Autodesk Inventor part; units mm, degrees
ref_plane "to_blackets_XY" through (0, 0, -4.5) normal (1, 0, 0) x (0, 0, -1)
ref_plane "to_blackets_YZ" through (0, 0, -4.5) normal (0, 0, -1) x (0, 1, 0)
ref_plane "to_blackets_ZX" through (0, 0, -4.5) normal (0, 1, 0) x (1, 0, 0)
sketch "_____1" plane through (0, 0, 0) normal (0, 0, 1) x (1, 0, 0)
  line L0 (-4.1, 2.7981) -> (-4.1, -2.7981)
  arc A0 (-4.1, -2.7981) -> (-4.0176, -2.9599) centre (-3.9, -2.7981) ccw
  line L1 (-4.0176, -2.9599) -> (-1.2622, -4.9618)
  arc A1 (-1.2622, -4.9618) -> (-1.1446, -5) centre (-1.1446, -4.8) ccw
  line L2 (-1.1446, -5) -> (-1, -5)
  arc A2 (-1, -5) -> (-0.8, -4.8) centre (-1, -4.8) ccw
  line L3 (-0.8, -4.8) -> (-0.8, -3)
  arc A3 (-0.7, -2.9) -> (-0.8, -3) centre (-0.7, -3) ccw
  line L4 (-0.7, -2.9) -> (-0.2, -2.9)
  arc A4 (-0.2, -2.9) -> (0, -2.7) centre (-0.2, -2.7) ccw
  line L5 (0, -2.7) -> (0, 2.7)
  arc A5 (0, 2.7) -> (-0.2, 2.9) centre (-0.2, 2.7) ccw
  line L6 (-0.2, 2.9) -> (-0.7, 2.9)
  arc A6 (-0.8, 3) -> (-0.7, 2.9) centre (-0.7, 3) ccw
  line L7 (-0.8, 3) -> (-0.8, 4.8)
  arc A7 (-0.8, 4.8) -> (-1, 5) centre (-1, 4.8) ccw
  line L8 (-1, 5) -> (-1.1446, 5)
  arc A8 (-1.1446, 5) -> (-1.2622, 4.9618) centre (-1.1446, 4.8) ccw
  line L9 (-1.2622, 4.9618) -> (-4.0176, 2.9599)
  arc A9 (-4.0176, 2.9599) -> (-4.1, 2.7981) centre (-3.9, 2.7981) ccw
extrude "Extrusion1" add sketch "_____1" against normal blind 14
sketch "_____2" plane through (0, 0, -4.5) normal (0, 0, 1) x (1, 0, 0)
  line L0 (0, 0) -> (-4.1, 0)
  line L1 (-4.1, 0) -> (-4.1, 2.5)
  line L2 (-4.1, 2.5) -> (-3.667, 2.067)
  line L3 (-3.667, 2.067) -> (-0.433, 2.067)
  line L4 (-0.433, 2.067) -> (0, 2.5)
  line L5 (0, 2.5) -> (0, 0)
  line L6 (0, 0) -> (-4.1, 0)
revolve "Revolution1" cut sketch "_____2" angle 360 about axis through (0, 0, -4.5) along (1, 0, 0)
thread "Thread1"
sketch "_____3" plane through (0, 0, -10.5) normal (0, 0, 1) x (1, 0, 0)
  line L0 (-3.05, 0) -> (-4.8, 0)
  line L1 (-4.8, 0) -> (-4.8, 1.75)
  line L2 (-4.8, 1.75) -> (-3.05, 1.75)
  line L3 (-3.05, 1.75) -> (-3.05, 0)
  line L4 (-3.05, 0) -> (-4.8, 0)
revolve "Revolution2" cut sketch "_____3" angle 360 about axis through (-3.05, 0, -10.5) along (1, 0, 0)
sketch "_____4" plane through (0, 0, -10.5) normal (0, 0, 1) x (1, 0, 0)
  line L0 (-3.05, 1.75) -> (-3.05, -1.75)
  arc A0 (-3.05, 1.75) -> (-3.05, -1.75) centre (-3.05, 0) ccw
  line L1 (-3.05, 1.75) -> (-3.05, -1.75)
revolve "Revolution3" add sketch "_____4" angle 360 about axis through (-3.05, 1.75, -10.5) along (0, 1, 0)
ref_plane "to_blackets_XY" through (0, 0, -4.5) normal (1, 0, 0) x (0, 0, -1)
ref_plane "to_blackets_YZ" through (0, 0, -4.5) normal (0, 0, -1) x (0, 1, 0)
ref_plane "to_blackets_ZX" through (0, 0, -4.5) normal (0, 1, 0) x (1, 0, 0)
ref_plane "to_bolt_XY" through (-4.1, 0, -4.5) normal (1, 0, 0) x (0, 0, -1)
ref_plane "to_bolt_YZ" through (-4.1, 0, -4.5) normal (0, 0, -1) x (0, 1, 0)
ref_plane "to_bolt_ZX" through (-4.1, 0, -4.5) normal (0, 1, 0) x (1, 0, 0)
ref_plane "to_frames_XY" through (-0.8, 0, -4.5) normal (1, 0, 0) x (0, 0, -1)
ref_plane "to_frames_YZ" through (-0.8, 0, -4.5) normal (0, 0, -1) x (0, 1, 0)
ref_plane "to_frames_ZX" through (-0.8, 0, -4.5) normal (0, 1, 0) x (1, 0, 0)
properties part number "HNTU5-5" material "ステンレス鋼"
Check sheet for the modelled part. Datum: model origin and axes. Units: mm. A direction names the side the tool comes from. Coordinates: 2 decimals unless noted, no trailing zeros. Order: outer loops, then holes, each group sorted by start corner. A loop starts at its lowest first (then second) coordinate and runs counter-clockwise, first axis right, second up. Notation, with made-up numbers: (-13, 41) -> (-8, 41) arc R15 cw to (-8, 65) -> close; hole circle Ø9 at (20.25, -0.75). An arc over 180 degrees is marked (long way). Write item = value, one per line. Start each with the question number.
1) Cross-section at B-B (y = 0). Enter the section's corners in (x, z).
2) Access from +Z, -Z, +X, -X, +Y, -Y to the whole of each face (thin tool, end or side, straight path). Record for faces 5 (the flat face through (-0.8, 4, -7)), 6 (the flat face through (-2.659, -3.947, -6.902)).
3) Cross-section at A-A (x = -3.3). Enter the section's corners in (y, z), then the cut area to 3 significant figures.
4) Material ranges on L1, parallel to Z at x = -1.5, y = 0; L2, parallel to Y at x = -0.35, z = -13.25; L3, parallel to X at y = -1, z = -0.5, recorded low to high.
5) Go/stop test with flat-tipped pins: P1, Ø1.4, axis at y = 4, z = -8.5, coming from the +X side; P2, Ø1, axis at x = -2, z = -4.5, coming from the +Y side; P3, Ø3.5, axis at y = 0, z = -4.5, coming from the +X side. Record where each tip stops, or that it passes through.
6) Mould release check, pull along Z, two halves, no side actions. Record for faces 1 (the flat face through (-2, 0, -14)), 2 (the flat face through (-2, 0, 0)), 3 (the flat face through (-0.8, -4, -7)), 4 (the cylindrical face through (-2.03, -0.27, -2.45)): +Z half, -Z half, draft (parallel to the pull), parting line (faces both ways), or undercut.
7) Cross-section at C-C (z = -4.5). Enter the section's corners in (x, y), then the cut area to 3 significant figures.
8) Cross-section at D-D (z = -10.5). Enter the section's corners in (x, y), then the cut area to 3 significant figures.
Ans:
q1.outline = (-4.1, -14) -> (0, -14) -> (0, -7) -> (-0.43, -6.57) -> (-3.67, -6.57) -> (-4.1, -7) -> (-4.1, -8.75) -> (-3.05, -8.75) arc R1.75 ccw to (-3.05, -12.25) -> (-4.1, -12.25) -> close; (-4.1, -2) -> (-3.67, -2.43) -> (-0.43, -2.43) -> (0, -2) -> (0, 0) -> (-4.1, 0) -> close
q2.face_5 = +Z, -Z, +X, +Y
q2.face_6 = +Z, -Z, -X, -Y
q3.outline = (-3.48, -14) -> (3.48, -14) -> (3.48, 0) -> (-3.48, 0) -> close; circle Ø3.46 at (0, -10.5); hole circle Ø4.13 at (0, -4.5); hole circle Ø3.5 at (0, -10.5)
q3.area = 83.9 mm²
q4.L1 = -14 to -6.57, -2.43 to 0
q4.L2 = -2.9 to 2.9
q4.L3 = -4.1 to 0
q5.P1 = -0.8
q5.P2 = 4.79
q5.P3 = through
q6.face_1 = -Z half
q6.face_2 = +Z half
q6.face_3 = draft
q6.face_4 = undercut
q7.outline = (-4.1, -2.8) arc R0.2 ccw to (-4.02, -2.96) -> (-1.26, -4.96) arc R0.2 ccw to (-1.14, -5) -> (-1, -5) arc R0.2 ccw to (-0.8, -4.8) -> (-0.8, -3) arc R0.1 cw to (-0.7, -2.9) -> (-0.2, -2.9) arc R0.2 ccw to (0, -2.7) -> (0, -2.5) -> (-0.43, -2.07) -> (-3.67, -2.07) -> (-4.1, -2.5) -> close; (-4.1, 2.5) -> (-3.67, 2.07) -> (-0.43, 2.07) -> (0, 2.5) -> (0, 2.7) arc R0.2 ccw to (-0.2, 2.9) -> (-0.7, 2.9) arc R0.1 cw to (-0.8, 3) -> (-0.8, 4.8) arc R0.2 ccw to (-1, 5) -> (-1.14, 5) arc R0.2 ccw to (-1.26, 4.96) -> (-4.02, 2.96) arc R0.2 ccw to (-4.1, 2.8) -> close
q7.area = 14.2 mm²
q8.outline = (-4.1, -2.8) arc R0.2 ccw to (-4.02, -2.96) -> (-1.26, -4.96) arc R0.2 ccw to (-1.14, -5) -> (-1, -5) arc R0.2 ccw to (-0.8, -4.8) -> (-0.8, -3) arc R0.1 cw to (-0.7, -2.9) -> (-0.2, -2.9) arc R0.2 ccw to (0, -2.7) -> (0, 2.7) arc R0.2 ccw to (-0.2, 2.9) -> (-0.7, 2.9) arc R0.1 cw to (-0.8, 3) -> (-0.8, 4.8) arc R0.2 ccw to (-1, 5) -> (-1.14, 5) arc R0.2 ccw to (-1.26, 4.96) -> (-4.02, 2.96) arc R0.2 ccw to (-4.1, 2.8) -> (-4.1, 1.75) -> (-3.05, 1.75) arc R1.75 ccw to (-3.05, -1.75) -> (-4.1, -1.75) -> close
q8.area = 32.7 mm²
